Here's how the part is built. I have some questions about the finished solid (model axes, mm). Face numbers are marked on the shaded views. A direction names the side the tool comes from. Coordinates: 2 decimals unless noted, no trailing zeros. Loops run counter-clockwise (first coordinate to the right, second up) from the corner with the lowest first, then second, coordinate; pieces in that order, holes last. Notation, with made-up numbers: (82, 2.25) -> (122, 2.25) arc R35 cw to (122, 41.25) -> close; hole circle Ø5 at (72.25, 89). An arc over 180 degrees is marked (long way). Answer as a JSON object with one key per item and string values. Group by question number.
Q1. I need wall thicknesses on line 1 (Y direction, x = -52.5, z = -6.5); line 2 (Y direction, x = -51, z = 2.25); line 3 (X direction, y = 20.5, z = -6.25). Which ranges of each line are inside material? Lowest first, please.
Q2. I want a section at B-B on x = -52.5. Write out the boundary of the cut face in (y, z), then the cut area to 3 significant figures.
Q3. I want a section at D-D on x = -45.75. Write out the boundary of the cut face in (y, z).
Q4. On a 3-axis mill with a long thin cutter (end or side, diameter ignored), from which of +Z, -Z, +X, -X, +Y, -Y can I reach the whole of each face in a straight line? I mean the marked faces 1, 2 and 3. Say none if no direction works.
Q5. I want a section at C-C on y = 20.5. Write out the boundary of the cut face in (x, z).
Q6. I want a section at A-A on z = -1.5. Write out the boundary of the cut face in (x, y).
Q7. I'm going to push flat-ended pins straight in: pin 1 (1.5 mm diameter, centred on x = -56, y = -3, fed in from -Z); pin 2 (0.8 mm diameter, centred on x = -47, z = -6.5, fed in from -Y); pin 3 (0.6 mm diameter, centred on x = -48.5, z = 6, fed in from +Y). Where does each tip first touch, or does it pass through?
```python
from build123d import *

# Parameters (mm, degrees)
CYLINDER100_R          = 1.5
CYLINDER100_DEPTH      = 10
CYLINDER103_R          = 1.5
CYLINDER103_DEPTH      = 5
CYLINDER104_R          = 1.5
CYLINDER104_DEPTH      = 10
CYLINDER102_R          = 3.5
CYLINDER102_DEPTH      = 5
BOX064_W               = 32
BOX064_H               = 13
BOX064_DEPTH           = 2
CYLINDER101_R          = 6.5
CYLINDER101_DEPTH      = 6
BOX063_W               = 23
BOX063_H               = 13
BOX063_DEPTH           = 24
CUT044_ROLL_ANGLE      = -90
CUT044_PLACEMENT_ANGLE = -90
CYLINDER086_R          = 1.4
CYLINDER086_DEPTH      = 4
BOX043_W               = 18
BOX043_H               = 29
BOX043_DEPTH           = 12.5
BOX044_W               = 18
BOX044_H               = 6
BOX044_DEPTH           = 17
BOX045_W               = 18
BOX045_H               = 6
BOX045_DEPTH           = 17
CYLINDER085_R          = 1.4
CYLINDER085_DEPTH      = 4
CYLINDER084_R          = 3.5
CYLINDER084_DEPTH      = 1
BOX042_W               = 16.5
BOX042_H               = 42
BOX042_DEPTH           = 14
CYLINDER021_R          = 1.4
CYLINDER021_DEPTH      = 2
CYLINDER022_R          = 1.4
CYLINDER022_DEPTH      = 2
BOX010_W               = 16
BOX010_H               = 32
BOX010_DEPTH           = 1
CYLINDER083_R          = 3.5
CYLINDER083_DEPTH      = 1


with BuildPart() as zylinder100:
    # Cylinder100 → Cylinder100 (new body)
    with BuildSketch(Plane(origin=(25.5, 6.5, 13), x_dir=(1, 0, 0), z_dir=(0, 0, 1))):
        Circle(CYLINDER100_R)
    extrude(amount=CYLINDER100_DEPTH)


with BuildPart() as zylinder103:
    # Cylinder103 → Cylinder103 (new body)
    with BuildSketch(Plane(origin=(16.5, 6.5, 30), x_dir=(1, 0, 0), z_dir=(0, 0, 1))):
        Circle(CYLINDER103_R)
    extrude(amount=CYLINDER103_DEPTH)


with BuildPart() as fusion061:
    # Cylinder104 → Cylinder104 (new body)
    with BuildSketch(Plane(origin=(-2.5, 6.5, 13), x_dir=(1, 0, 0), z_dir=(0, 0, 1))):
        Circle(CYLINDER104_R)
    extrude(amount=CYLINDER104_DEPTH)

    # Fusion061: union Zylinder100, Zylinder103
    add(zylinder100.part)
    add(zylinder103.part)


with BuildPart() as zylinder102:
    # Cylinder102 → Cylinder102 (new body)
    with BuildSketch(Plane(origin=(16.5, 6.5, 29), x_dir=(1, 0, 0), z_dir=(0, 0, 1))):
        Circle(CYLINDER102_R)
    extrude(amount=CYLINDER102_DEPTH)


with BuildPart() as obj1:
    # Box064 → Box064 (new body)
    with BuildSketch(Plane(origin=(-4.5, 0, 18), x_dir=(1, 0, 0), z_dir=(0, 0, 1))):
        with Locations((16, 6.5)):
            Rectangle(BOX064_W, BOX064_H)
    extrude(amount=BOX064_DEPTH)


with BuildPart() as zylinder101:
    # Cylinder101 → Cylinder101 (new body)
    with BuildSketch(Plane(origin=(16.5, 6.5, 23), x_dir=(1, 0, 0), z_dir=(0, 0, 1))):
        Circle(CYLINDER101_R)
    extrude(amount=CYLINDER101_DEPTH)


with BuildPart() as servo3_mask001:
    # Box063 → Box063 (new body)
    with BuildSketch(Plane.XY.offset(-1)):
        with Locations((11.5, 6.5)):
            Rectangle(BOX063_W, BOX063_H)
    extrude(amount=BOX063_DEPTH)

    # Fusion060: union Zylinder102, obj1, Zylinder101
    add(zylinder102.part)
    add(obj1.part)
    add(zylinder101.part)

    # Cut044: cut Fusion061
    add(fusion061.part, mode=Mode.SUBTRACT)


with BuildPart() as servo3_mask001_1:
    # Cut044 roll: moved
    add(servo3_mask001.part.rotate(Axis((0, 0, 0), (1, 0, 0)), CUT044_ROLL_ANGLE))


with BuildPart() as servo3_mask001_2:
    # Cut044 placement: moved
    add(servo3_mask001_1.part.moved(Location((-49.5, 16.5, 5))).rotate(Axis((-49.5, 16.5, 5), (0, 0, 1)), CUT044_PLACEMENT_ANGLE))


with BuildPart() as zylinder086:
    # Cylinder086 → Cylinder086 (new body)
    with BuildSketch(Plane(origin=(-52.5, 20.5, -9.5), x_dir=(1, 0, 0), z_dir=(0, 0, 1))):
        Circle(CYLINDER086_R)
    extrude(amount=CYLINDER086_DEPTH)


with BuildPart() as obj2:
    # Box043 → Box043 (new body)
    with BuildSketch(Plane(origin=(-61.5, -14.5, -8), x_dir=(1, 0, 0), z_dir=(0, 0, 1))):
        with Locations((9, 14.5)):
            Rectangle(BOX043_W, BOX043_H)
    extrude(amount=BOX043_DEPTH)


with BuildPart() as obj3:
    # Box044 → Box044 (new body)
    with BuildSketch(Plane(origin=(-61.5, -22, -7), x_dir=(1, 0, 0), z_dir=(0, 0, 1))):
        with Locations((9, 3)):
            Rectangle(BOX044_W, BOX044_H)
    extrude(amount=BOX044_DEPTH)


with BuildPart() as obj4:
    # Box045 → Box045 (new body)
    with BuildSketch(Plane(origin=(-61.5, 16, -7), x_dir=(1, 0, 0), z_dir=(0, 0, 1))):
        with Locations((9, 3)):
            Rectangle(BOX045_W, BOX045_H)
    extrude(amount=BOX045_DEPTH)


with BuildPart() as fusion093:
    # Cylinder085 → Cylinder085 (new body)
    with BuildSketch(Plane(origin=(-52.5, -20.5, -9.5), x_dir=(1, 0, 0), z_dir=(0, 0, 1))):
        Circle(CYLINDER085_R)
    extrude(amount=CYLINDER085_DEPTH)

    # Fusion047: union Zylinder086, obj2, obj3, obj4
    add(zylinder086.part)
    add(obj2.part)
    add(obj3.part)
    add(obj4.part)

    # Fusion093: union Servo3_mask001
    add(servo3_mask001_2.part)


with BuildPart() as zylinder084:
    # Cylinder084 → Cylinder084 (new body)
    with BuildSketch(Plane(origin=(-52.5, 20.5, -8), x_dir=(1, 0, 0), z_dir=(0, 0, 1))):
        Circle(CYLINDER084_R)
    extrude(amount=CYLINDER084_DEPTH)


with BuildPart() as obj5:
    # Box042 → Box042 (new body)
    with BuildSketch(Plane(origin=(-60.5, -21, -8), x_dir=(1, 0, 0), z_dir=(0, 0, 1))):
        with Locations((8.25, 21)):
            Rectangle(BOX042_W, BOX042_H)
    extrude(amount=BOX042_DEPTH)


with BuildPart() as zylinder021:
    # Cylinder021 → Cylinder021 (new body)
    with BuildSketch(Plane(origin=(16.5, 10, -26.5), x_dir=(1, 0, 0), z_dir=(0, 0, 1))):
        Circle(CYLINDER021_R)
    extrude(amount=CYLINDER021_DEPTH)


with BuildPart() as zylinder022:
    # Cylinder022 → Cylinder022 (new body)
    with BuildSketch(Plane(origin=(16.5, -10, -26.5), x_dir=(1, 0, 0), z_dir=(0, 0, 1))):
        Circle(CYLINDER022_R)
    extrude(amount=CYLINDER022_DEPTH)


with BuildPart() as fusion009:
    # Box010 → Box010 (new body)
    with BuildSketch(Plane(origin=(8.5, -16, -27.5), x_dir=(1, 0, 0), z_dir=(0, 0, 1))):
        with Locations((8, 16)):
            Rectangle(BOX010_W, BOX010_H)
    extrude(amount=BOX010_DEPTH)

    # Fusion009: union Zylinder021, Zylinder022
    add(zylinder021.part)
    add(zylinder022.part)


with BuildPart() as fusion009_1:
    # Fusion009 placement: moved
    add(fusion009.part.moved(Location((-69, 0, 32.5))))


with BuildPart() as cut082:
    # Cylinder083 → Cylinder083 (new body)
    with BuildSketch(Plane(origin=(-52.5, -20.5, -8), x_dir=(1, 0, 0), z_dir=(0, 0, 1))):
        Circle(CYLINDER083_R)
    extrude(amount=CYLINDER083_DEPTH)

    # Fusion046: union Zylinder084, obj5, Fusion009
    add(zylinder084.part)
    add(obj5.part)
    add(fusion009_1.part)

    # Cut082: cut Fusion093
    add(fusion093.part, mode=Mode.SUBTRACT)


with BuildPart() as cut082_1:
    # Cut082 placement: moved
    add(cut082.part.moved(Location((0, 0, 1))))


solid = cut082_1.part
```
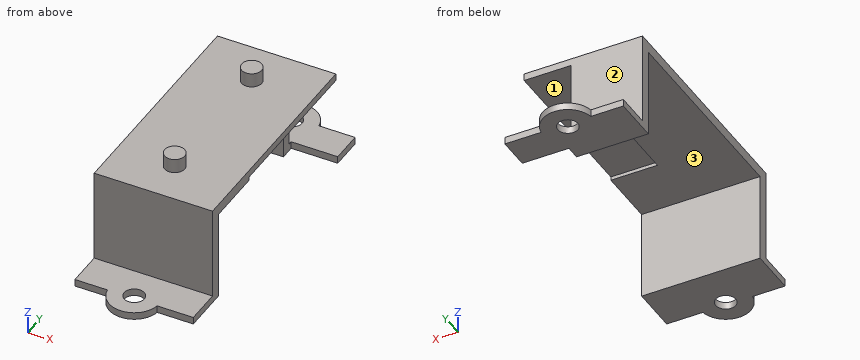
Result set:
{
 "1": {"line 1": "y = -24 to -21.9, -19.1 to -14.5, 14.5 to 19.1, 21.9 to 24", "line 2": "y = -16 to -14.5, 14.5 to 16", "line 3": "x = -60.5 to -53.9, -51.1 to -44"},
 "2": {"outline": "(-24, -7) -> (-21.9, -7) -> (-21.9, -6) -> (-24, -6) -> close; (-19.1, -7) -> (-14.5, -7) -> (-14.5, 5.5) -> (14.5, 5.5) -> (14.5, -7) -> (19.1, -7) -> (19.1, -6) -> (16, -6) -> (16, 7) -> (11.4, 7) -> (11.4, 9) -> (8.6, 9) -> (8.6, 7) -> (-8.6, 7) -> (-8.6, 9) -> (-11.4, 9) -> (-11.4, 7) -> (-16, 7) -> (-16, -6) -> (-19.1, -6) -> close; (21.9, -7) -> (24, -7) -> (24, -6) -> (21.9, -6) -> close", "area": "107 mm²"},
 "3": {"outline": "(-21, -7) -> (-14.5, -7) -> (-14.5, 5.5) -> (-6.5, 5.5) -> (-6.5, 6) -> (16, 6) -> (16, 7) -> (-16, 7) -> (-16, -6) -> (-21, -6) -> close; (16.5, -7) -> (21, -7) -> (21, -6) -> (16.5, -6) -> close"},
 "4": {"face 1": "-Z, +X, +Y", "face 2": "+Z, +X, -X, +Y", "face 3": "-Z, +X, -X"},
 "5": {"outline": "(-60.5, -7) -> (-53.9, -7) -> (-53.9, -6) -> (-60.5, -6) -> close; (-51.1, -7) -> (-44, -7) -> (-44, -6) -> (-51.1, -6) -> close"},
 "6": {"outline": "(-60.5, -16) -> (-44, -16) -> (-44, -14.5) -> (-60.5, -14.5) -> close; (-60.5, 14.5) -> (-50.5, 14.5) -> (-50.5, 16) -> (-60.5, 16) -> close"},
 "7": {"pin 1": "stops at z = 5.5", "pin 2": "stops at y = -21", "pin 3": "stops at y = 16"}
}
